from build123d import *

# Parameters (mm, degrees)
F0_W      = 152.4
F0_H      = 152.399992557
F1_DEPTH  = 152.4
F2_R      = 8.5037572656
F3_DEPTH  = 12.7
F4_R      = 7.0073319603
F4_R_2    = 6.9501235212
F4_R_3    = 6.7658122989
F5_DEPTH  = 12.7
F6_R      = 7.0073351943
F6_R_2    = 6.9545325537
F7_DEPTH  = 12.7
F8_R      = 7.0452123399
F8_R_2    = 7.0168230938
F9_DEPTH  = 12.7
F10_R     = 7.0828869948
F10_R_2   = 7.1489340482
F10_R_3   = 7.2408196542
F11_DEPTH = 12.7
F12_R     = 6.6966018478
F12_R_2   = 6.8804301319
F12_R_3   = 6.7065356098
F12_R_4   = 6.6881507526
F12_R_5   = 6.8147907528
F12_R_6   = 6.6567393836
F13_DEPTH = 12.7
F14_R     = 7.0168186878
F14_R_2   = 6.8827909579
F14_R_3   = 7.0168182521
F14_R_4   = 6.7263512429
F15_DEPTH = 12.7


with BuildPart() as f1:
    # F0 (on Front) → F1 (new body)
    with BuildSketch(Plane.XZ):
        with Locations((0.2630501986, -0.2443604171)):
            Rectangle(F0_W, F0_H)
    extrude(amount=F1_DEPTH)

    # F2 (on face) → F3 (cut)
    with BuildSketch(Plane.XY.offset(75.9556358614)):
        with Locations((0, -76.037876308)):
            Circle(F2_R)
    extrude(amount=-F3_DEPTH, mode=Mode.SUBTRACT)

    # F4 (on face) → F5 (cut)
    with BuildSketch(Plane(origin=(0, 0, 0), x_dir=(-1, 0, 0), z_dir=(0, 1, 0))):
        with Locations((67.3541128635, 63.7721791863)):
            Circle(F4_R)
        with Locations((64.4358173013, -62.6201629639)):
            Circle(F4_R_2)
        with Locations((-66.1580115557, -63.6519268155)):
            Circle(F4_R_3)
    extrude(amount=-F5_DEPTH, mode=Mode.SUBTRACT)

    # F6 (on face) → F7 (cut)
    with BuildSketch(Plane(origin=(0, 0, 0), x_dir=(-1, 0, 0), z_dir=(0, 1, 0))):
        with Locations((-66.8875873089, 64.2880648375)):
            Circle(F6_R)
        Circle(F6_R_2)
    extrude(amount=-F7_DEPTH, mode=Mode.SUBTRACT)

    # F8 (on face) → F9 (cut)
    with BuildSketch(Plane.XZ.offset(152.4)):
        with Locations((-55.3161352873, 56.7846298218)):
            Circle(F8_R)
        with Locations((54.8496097326, -60.6768615544)):
            Circle(F8_R_2)
    extrude(amount=-F9_DEPTH, mode=Mode.SUBTRACT)

    # F10 (on face) → F11 (cut)
    with BuildSketch(Plane(origin=(-75.9369498014, 0, 0), x_dir=(0, -1, 0), z_dir=(-1, 0, 0))):
        with Locations((15.1184033602, -60.3120736778)):
            Circle(F10_R)
        with Locations((76.037876308, 0)):
            Circle(F10_R_2)
        with Locations((135.1334154606, 65.9043118358)):
            Circle(F10_R_3)
    extrude(amount=-F11_DEPTH, mode=Mode.SUBTRACT)

    # F12 (on face) → F13 (cut)
    with BuildSketch(Plane(origin=(0, 0, -76.4443566957), x_dir=(1, 0, 0), z_dir=(0, 0, -1))):
        with Locations((58.1326968968, 17.6719166338)):
            Circle(F12_R)
        with Locations((0, 18.4014886618)):
            Circle(F12_R_2)
        with Locations((-54.5865595341, 19.4958504289)):
            Circle(F12_R_3)
        with Locations((0, 140.2404308319)):
            Circle(F12_R_4)
        with Locations((-57.8696429729, 140.9700065851)):
            Circle(F12_R_5)
        with Locations((59.2270568013, 141.6995823383)):
            Circle(F12_R_6)
    extrude(amount=-F13_DEPTH, mode=Mode.SUBTRACT)

    # F14 (on face) → F15 (cut)
    with BuildSketch(Plane.YZ.offset(76.4630501986)):
        with Locations((-10.0113833323, 63.7155920267)):
            Circle(F14_R)
        with Locations((-12.5648928806, -60.6768615544)):
            Circle(F14_R_2)
        with Locations((-143.5235142708, 64.8099482059)):
            Circle(F14_R_3)
        with Locations((-143.5235142708, -66.5134564042)):
            Circle(F14_R_4)
    extrude(amount=-F15_DEPTH, mode=Mode.SUBTRACT)


solid = f1.part
CAD build for the part. Positions are in the model's coordinates, mm. A direction names the side the tool comes from. Coordinates: 2 decimals unless noted, no trailing zeros. Loops run counter-clockwise (first coordinate to the right, second up) from the corner with the lowest first, then second, coordinate; pieces in that order, holes last. Notation, with made-up numbers: (89.25, 55) - (109.25, 55) arc R14 cw to (109.25, 74) - close; hole circle Ø1 at (68.5, 88). An arc over 180 degrees is marked (long way). Write item = value, one per line. Start each with the question number.
Q1. Pull direction Y, two halves, no side cores. Call faces 1 (the flat face through (-55, -20, -63.744)), 2 (the flat face through (-67, -12.7, 64)), 3 (the flat face through (76.463, -75, -1)): pulls with the +Y half, pulls with the -Y half, needs draft (parallel to the pull), parting line crosses it, or undercut.
Q2. Cut at A-A, the plane x = 0. List the corners of the cut face in (y, z), then the cut area to 3 significant figures.
Q3. Which spindle directions (+Z, -Z, +X, -X, +Y, -Y) get a long thin tool onto all of the face, cutting with end or side? Do faces 4 (the flat face through (58, -18, -63.744)), 5 (the cylindrical face through (70.202, -144.399, -59.844)), 6 (the cylindrical face through (53.94, -146.14, -53.72)). Say none if no direction does.
Q4. Drill centre lines: L1, parallel to Y at x = 0, z = -66.25; L2, parallel to Y at x = 0, z = 68; L3, parallel to Z at x = -3, y = -77. Where is each one in solid material? Low to high.
Q5. Cut at B-B, the plane z = 0. List the corners of the cut face in (x, y).
Q6. Flat gauge pins, fed straight in: pin 1 Ø6.5 at (x, y) = (60.5, -20) entering from -Z; pin 2 Ø11.5 at (x, z) = (-55.32, 56.78) entering from -Y; pin 3 Ø4 at (y, z) = (-144, 68) entering from +X. Where does each tip first touch, or does it go through?
Computed:
q1.face_1 = undercut
q1.face_2 = pulls with the +Y half
q1.face_3 = needs draft
q2.outline = (-152.4, -76.44) - (-146.93, -76.44) - (-146.93, -63.74) - (-133.55, -63.74) - (-133.55, -76.44) - (-25.28, -76.44) - (-25.28, -63.74) - (-11.52, -63.74) - (-11.52, -76.44) - (0, -76.44) - (0, -6.95) - (-12.7, -6.95) - (-12.7, 6.95) - (0, 6.95) - (0, 75.96) - (-67.53, 75.96) - (-67.53, 63.26) - (-84.54, 63.26) - (-84.54, 75.96) - (-152.4, 75.96) - close
q2.area = 22,500 mm²
q3.face_4 = -Z
q3.face_5 = +X
q3.face_6 = -Y
q4.L1 = -152.4 to -146.93, -133.55 to -25.28, -11.52 to 0
q4.L2 = -152.4 to -84.54, -67.53 to 0
q4.L3 = -76.44 to 63.26
q5.outline = (-75.94, -152.4) - (76.46, -152.4) - (76.46, 0) - (6.95, 0) - (6.95, -12.7) - (-6.95, -12.7) - (-6.95, 0) - (-75.94, 0) - (-75.94, -68.89) - (-63.24, -68.89) - (-63.24, -83.19) - (-75.94, -83.19) - close
q6.pin_1 = -63.74
q6.pin_2 = -139.7
q6.pin_3 = 63.76
